Geometry: final body of the model. Coordinates: model frame, mm. Coordinates: 2 decimals unless noted, no trailing zeros. Loops run counter-clockwise (first coordinate to the right, second up) from the corner with the lowest first, then second, coordinate; pieces in that order, holes last. Notation, with made-up numbers: M -19.75,13 L 17.25,13 A10 cw 17.25,32 Z; hole C -22,16.5 d7. An arc over 180 degrees is marked long. Write each question's results on one line, items separated by ' | '. Start each with the question number.
Autodesk Inventor part; units mm, degrees
ref_plane "YZ Plane" through (0, 0, 0) normal (1, 0, 0) x (0, 1, 0)
ref_plane "XZ Plane" through (0, 0, 0) normal (0, 1, 0) x (-1, 0, 0)
ref_plane "XY Plane" through (0, 0, 0) normal (0, 0, 1) x (1, 0, 0)
sketch "Sketch1" plane through (0, 0, 0) normal (0, 1, 0) x (-1, 0, 0)
  line L0 (38.1, -177.8) -> (38.1, -101.6)
  line L1 (38.1, -101.6) -> (-38.1, -101.6)
  line L2 (-38.1, -101.6) -> (-38.1, -177.8)
  line L3 (38.1, 177.8) -> (38.1, 101.6)
  line L4 (38.1, 101.6) -> (-38.1, 101.6)
  line L5 (-38.1, 101.6) -> (-38.1, 177.8)
  line L6 (177.8, 38.1) -> (101.6, 38.1)
  line L7 (101.6, 38.1) -> (101.6, -38.1)
  line L8 (101.6, -38.1) -> (177.8, -38.1)
  line L9 (-101.6, -38.1) -> (-177.8, -38.1)
  line L10 (-101.6, -38.1) -> (-101.6, 38.1)
  line L11 (-101.6, 38.1) -> (-177.8, 38.1)
  arc A0 (38.1, -177.8) -> (177.8, -38.1) centre (0, 0) ccw
  arc A1 (-177.8, -38.1) -> (-38.1, -177.8) centre (0, 0) ccw
  arc A2 (177.8, 38.1) -> (38.1, 177.8) centre (-0.0019, -0.0019) ccw
  arc A3 (-38.1, 177.8) -> (-177.8, 38.1) centre (0.0019, -0.0019) ccw
  dimension "d0" = 76.2
  dimension "d2" = 76.2
  dimension "d3" = 76.2
  dimension "d4" = 76.2
  dimension "d5" = 76.2
  dimension "d6" = 76.2
  dimension "d7" = 101.6
  dimension "d8" = 101.6
  dimension "d9" = 38.1
  dimension "d10" = 38.1
  dimension "d11" = 76.2
  dimension "d12" = 76.2
  dimension "d13" = 76.2
  dimension "d14" = 101.6
  dimension "d15" = 38.1
  dimension "d16" = 76.2
  dimension "d17" = 76.2
  dimension "d18" = 76.2
  dimension "d19" = 101.6
  dimension "d20" = 38.1
  dimension "d23" = 0
  dimension "d25" = 0
  dimension "d26" = 181.8363
  dimension "d27" = 181.8363
  dimension "d28" = 181.8386
  dimension "d30" = 181.8386
extrude "Plate1" add sketch "Sketch1" along normal blind 3.175
sketch "Sketch2" plane through (0, 3.175, 0) normal (0, 1, 0) x (1, 0, 0)
  arc A0 (-177.8, -38.1) -> (-38.1, -177.8) centre (0.0019, 0.0019) ccw
  arc A1 (38.1, -177.8) -> (177.8, -38.1) centre (-0.0019, 0.0019) ccw
  line L0 (-25.4019, -25.3981) -> (25.3981, -25.3981) construction
  line L1 (25.3981, -25.3981) -> (25.3981, 25.4019) construction
  line L2 (25.3981, 25.4019) -> (-25.4019, 25.4019) construction
  line L3 (-25.4019, 25.4019) -> (-25.4019, -25.3981) construction
  dimension "d50" = 50.8
  dimension "d52" = 50.8
  dimension "d53" = 25.4
  dimension "d54" = 25.4
hole "Hole2" at (-25.4019, 3.175, -25.4019) at (25.3981, 3.175, -25.4019) at (25.3981, 3.175, 25.3981) at (-25.4019, 3.175, 25.3981) direction (0, -1, 0) diameter 6.35 depth 3.175
sketch "Sketch3" plane through (0, 3.175, 0) normal (0, 1, 0) x (1, 0, 0)
  arc A0 (177.8, 38.1) -> (38.1, 177.8) centre (0, 0) ccw
hole "Hole3" at (0, 3.175, 0) direction (0, -1, 0) diameter 6.35 depth 3.175 tip angle 118
equation "\"d2\" = d0"
equation "\"d3\" = d0"
equation "\"d4\" = d0"
equation "\"d5\" = d6"
equation "\"d11\" = d0"
equation "\"d12\" = d0"
equation "\"d13\" = d6"
equation "\"d16\" = d6"
equation "\"d17\" = d0"
equation "\"d18\" = d0"
equation "\"d60\" = Thickness"
equation "\"d67\" = Thickness"
equation "\"BendRadius\" = Thickness"
equation "\"BendReliefWidth\" = Thickness"
equation "\"BendReliefDepth\" = 0.5 * Thickness"
equation "\"CornerReliefSize\" = 4 * Thickness"
equation "\"MinimumRemnant\" = 2 * Thickness"
equation "\"TransitionRadius\" = BendRadius"
equation "\"JacobiRadiusSize\" = BendRadius"
equation "\"GapSize\" = Thickness"
equation "\"d31\" = BendRadius"
properties part number "TopCover"
Item 1: Section D-D, the plane z = -64.5. Return loops of the section in (x, y) (3 decimals), plus the area to 3 significant figures.
Item 2: Ray query, L1, parallel to X at y = 0.7, z = 0 (3 decimals); L2, parallel to Z at x = -11, y = 1.2; L3, parallel to Z at x = -129.5, y = 1.1. Return the intervals inside material, ascending. Write a range as [from, to].
Item 3: Section A-A, the plane x = -108.5. Return loops of the section in (y, z) (3 decimals).
Item 4: Contact query for flat-ended pins moving along their axis: P1, Ø8.5, axis at x = 25.4, z = 25.4, coming from the -Y side; P2, Ø1.6, axis at x = 139, y = 2, coming from the -Z side; P3, Ø1.6, axis at x = 145, y = 2, coming from the +Z side; P4, Ø1, axis at x = 17, y = 2, coming from the +Z side. Output: stop coordinate, or through.
Item 5: Section B-B, the plane y = 2. Return loops of the section in (x, z) (3 decimals).
Item 6: Section C-C, the plane x = 128.5. Return loops of the section in (y, z) (3 decimals), plus the area to 3 significant figures.
Solutions:
1) outline: M -170.012,0 L 170.012,0 L 170.012,3.175 L -170.012,3.175 Z | area: 1,080 mm²
2) L1: x = [-101.6, -3.175], [3.175, 101.6] | L2: z = [-101.6, 101.6] | L3: z = [-127.65, -38.1], [38.1, 127.65]
3) outline: M 0,-145.918 L 3.175,-145.918 L 3.175,-38.1 L 0,-38.1 Z; M 0,38.1 L 3.175,38.1 L 3.175,145.918 L 0,145.918 Z
4) P1: stops at y = 0 | P2: stops at z = -118.17 | P3: stops at z = 110.77 | P4: stops at z = 101.6
5) outline: M -177.8,-38.1 A181.836 ccw -38.1,-177.8 L -38.1,-101.6 L 38.1,-101.6 L 38.1,-177.8 A181.836 ccw 177.8,-38.1 L 101.6,-38.1 L 101.6,38.1 L 177.8,38.1 A181.839 ccw 38.1,177.8 L 38.1,101.6 L -38.1,101.6 L -38.1,177.8 A181.839 ccw -177.8,38.1 L -101.6,38.1 L -101.6,-38.1 Z; hole C -25.402,-25.402 d6.35; hole C -25.402,25.398 d6.35; hole C 0,0 d6.35; hole C 25.398,-25.402 d6.35; hole C 25.398,25.398 d6.35
6) outline: M 0,-128.655 L 3.175,-128.655 L 3.175,-38.1 L 0,-38.1 Z; M 0,38.1 L 3.175,38.1 L 3.175,128.655 L 0,128.655 Z | area: 575 mm²
